Can you work these out from the model? Positions are in its coordinate system, mm. A direction names the side the tool comes from. Give positions to 0.01 mm unless a question says otherwise; leave off trailing zeros. Order: outer loops, then holes, each group sorted by start corner. A loop starts at its lowest first (then second) coordinate and runs counter-clockwise, first axis right, second up. Notation, with made-up numbers: (-1.75, 51.5) -> (48.25, 51.5) arc R20 cw to (48.25, 55.5) -> close; hole circle Ø10 at (-3.5, 4.5). An arc over 180 degrees is marked (long way). Answer as a JSON object with one key per item and string values.
```python
from build123d import *

# Parameters (mm, degrees)
EXTRUDE_1_DEPTH     = 48
CUT_EXTRUDE_1_DEPTH = 48
FILLET_1_R          = 2


with BuildPart() as part:
    # 草圖1 → 填料-伸長1 (new body)
    with BuildSketch(Plane.XY):
        with BuildLine():
            Line((0, 0), (8, 0))
            Line((8, 0), (8, 47))
            ThreePointArc((8, 47), (25, 64), (42, 47))
            Line((42, 47), (42, 0))
            Line((42, 0), (110, 0))
            Line((110, 0), (110, 15))
            Line((110, 15), (50, 15))
            Line((50, 15), (50, 47))
            ThreePointArc((50, 47), (25, 72), (0, 47))
            Line((0, 47), (0, 0))
        make_face()
    extrude(amount=-EXTRUDE_1_DEPTH)

    # 草圖2 → 除料-伸長1 (cut)
    with BuildSketch(Plane(origin=(0, 15, 0), x_dir=(1, 0, 0), z_dir=(0, 1, 0))):
        with BuildLine():
            Line((74, 0), (74, 16))
            Line((74, 16), (80, 16))
            Line((80, 16), (80, 28))
            ThreePointArc((80, 28), (90, 38), (100, 28))
            Line((100, 28), (100, 16))
            Line((100, 16), (110, 16))
            Line((110, 16), (110, 0))
            Line((110, 0), (74, 0))
        make_face()
    extrude(amount=-CUT_EXTRUDE_1_DEPTH, mode=Mode.SUBTRACT)

    # 圓角1
    fillet_1_edges = [part.edges().sort_by_distance(p)[0] for p in [
        (50, 15, -24),
    ]]
    fillet(fillet_1_edges, radius=FILLET_1_R)


solid = part.part
```
1. Please list where these lines run through material, in increasing order: L1, parallel to X at y = 4.5, z = -6; L2, parallel to X at y = 27, z = -8; L3, parallel to Y at x = 62, z = -34.5.
Worked answers:
{"L1": "0 to 8, 42 to 74", "L2": "0 to 8, 42 to 50", "L3": "0 to 15"}
2. If we mould it in two halves opening along X, with no side actions, what happens to faces 1 (the face through (42, 24, -24)), 2 (the face through (74, 8, -8)), 3 (the face through (25.55, 71.994, -23.664))? For each: +X half, -X half, draft (parallel to the pull), parting line (faces both ways), or undercut.
Worked answers:
{"face 1": "undercut", "face 2": "+X half", "face 3": "parting line"}
3. Will these pins go through, and if not, where does the flat tip stop? pin 1 Ø6 at (x, z) = (12.5, -11.5) entering from -Y; pin 2 Ø12 at (y, z) = (10.5, -6.5) entering from +X; pin 3 Ø6.5 at (x, y) = (78, 5) entering from +Z.
Worked answers:
{"pin 1": "y = 53.98", "pin 2": "x = 74", "pin 3": "z = -16"}
4. If we section it at B-B on z = -6: Please give me the cut outline in (x, y), then the cut area to 3 significant figures.
Worked answers:
{"outline": "(0, 0) -> (8, 0) -> (8, 47) arc R17 cw to (42, 47) -> (42, 0) -> (74, 0) -> (74, 15) -> (52, 15) arc R2 cw to (50, 17) -> (50, 47) arc R25 ccw to (0, 47) -> close", "area": "1,640 mm²"}
5. If we section it at A-A on y = 30.5: Please give me the cut outline in (x, z).
Worked answers:
{"outline": "(0, -48) -> (8, -48) -> (8, 0) -> (0, 0) -> close; (42, -48) -> (50, -48) -> (50, 0) -> (42, 0) -> close"}
6. For faces 4 (the face through (50, 32, -24)), 5 (the face through (80, 8, -22)), 6 (the face through (105, 8, -16)), 7 (the face through (8, 23, -24)), which set-ups out of +Z, -Z, +X, -X, +Y, -Y let a thin tool reach every point of the face, with its end or its side?
Worked answers:
{"face 4": "+Z, -Z, +X, +Y", "face 5": "+Z, +Y, -Y", "face 6": "+Z, +X, +Y, -Y", "face 7": "+Z, -Z, -Y"}
7. If we section it at D-D on x = 90: Please give me the cut outline in (y, z), then the cut area to 3 significant figures.
Worked answers:
{"outline": "(0, -48) -> (15, -48) -> (15, -38) -> (0, -38) -> close", "area": "150 mm²"}
8. If we section it at C-C on z = -17.5: Please give me the cut outline in (x, y).
Worked answers:
{"outline": "(0, 0) -> (8, 0) -> (8, 47) arc R17 cw to (42, 47) -> (42, 0) -> (80, 0) -> (80, 15) -> (52, 15) arc R2 cw to (50, 17) -> (50, 47) arc R25 ccw to (0, 47) -> close; (100, 0) -> (110, 0) -> (110, 15) -> (100, 15) -> close"}
